Design review of the part shown in the three views and the two pictorial views. Dimensions are in mm from the part's minimum x, y and z. A direction names the side the tool comes from. Give positions to 0.01 mm unless a question says otherwise; leave off trailing zeros. Order: outer loops, then holes, each group sorted by start corner. A loop starts at its lowest first (then second) coordinate and runs counter-clockwise, first axis right, second up.
Item 1: Consider section B-B (x = 10.75). Give the boundary of the cut face in (y, z), plus the area to 3 significant figures.
Item 2: For P1, Ø1.9, axis at x = 7.5, z = 6, coming from the -Y side, flat-tipped, find the tip position at first contact; note if it passes through.
Item 3: The part is to be moulded in two halves that separate along X. For the marked faces 1, 2 and 3, say which applies: released by +X, released by -X, zero draft, split by the parting line, or undercut.
Item 4: Machinability: for the marked faces 4 and 5, which of the approach directions +Z, -Z, +X, -X, +Y, -Y give a long, thin tool a straight path to every point of the face, cutting with its end or side? Answer none if there is none.
Item 5: For probe 1 along Y at (x, z) = (10.5, 4.5); probe 2 along X at (y, z) = (5.5, 6); probe 3 along Y at (x, z) = (7.75, 3.25), list the stretches that pass through material, from the lowest coordinate up.
Item 6: Consider section D-D (x = 5.5). Give the boundary of the cut face in (y, z) (1 decimal).
Item 7: Consider section C-C (y = 2). Give the boundary of the cut face in (x, z), plus the area to 3 significant figures.
Item 8: Consider section A-A (z = 6). Give the boundary of the cut face in (x, y) (1 decimal).
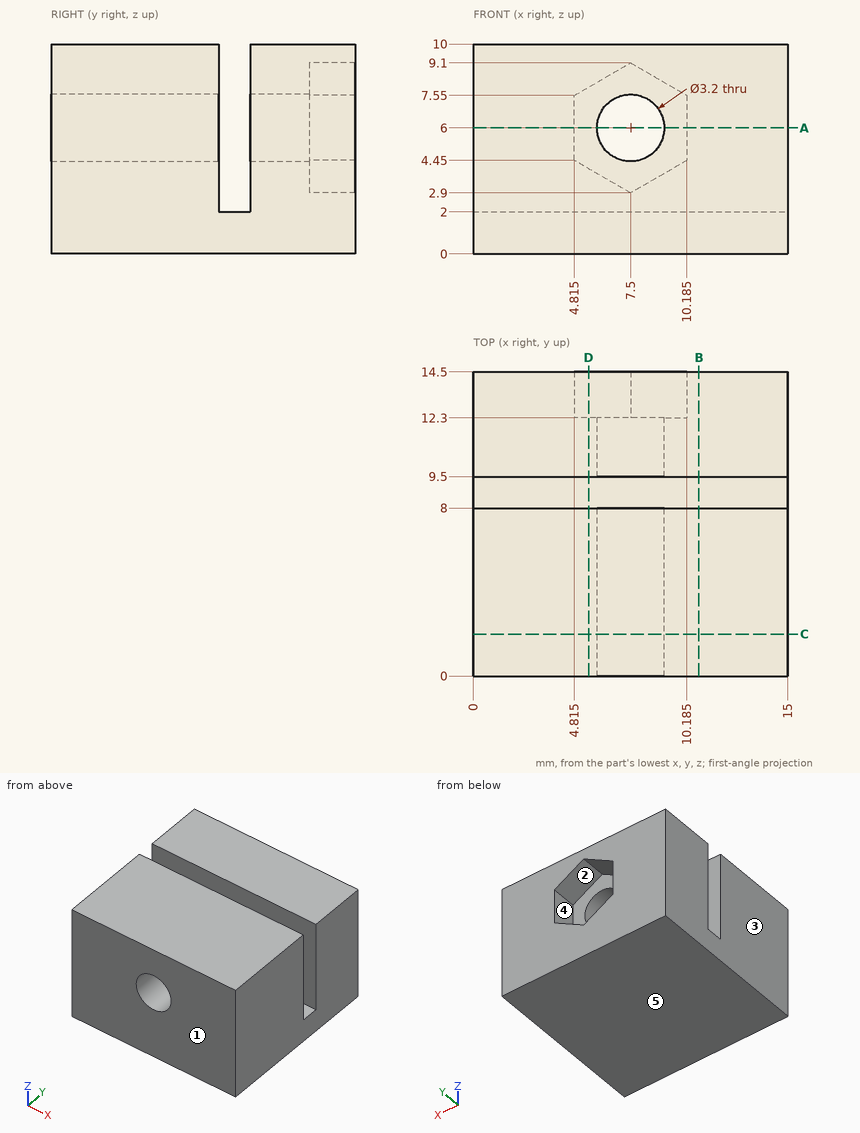
Resolved:
1. outline: (0, 0) - (14.5, 0) - (14.5, 10) - (9.5, 10) - (9.5, 2) - (8, 2) - (8, 10) - (0, 10) - close
1. area: 133 mm2
2. P1: passes through
3. face 1: zero draft
3. face 2: undercut
3. face 3: released by -X
4. face 4: +Y
4. face 5: -Z, +X, -X, +Y, -Y
5. probe 1: y = 0 to 8, 9.5 to 14.5
5. probe 2: x = 0 to 5.9, 9.1 to 15
5. probe 3: y = 0 to 8, 9.5 to 12.3
6. outline: (0, 0) - (14.5, 0) - (14.5, 4.1) - (12.3, 4.1) - (12.3, 7.9) - (14.5, 7.9) - (14.5, 10) - (9.5, 10) - (9.5, 2) - (8, 2) - (8, 10) - (0, 10) - close
7. outline: (0, 0) - (15, 0) - (15, 10) - (0, 10) - close; hole circle Ø3.2 at (7.5, 6)
7. area: 142 mm2
8. outline: (0, 0) - (5.9, 0) - (5.9, 8) - (0, 8) - close; (0, 9.5) - (5.9, 9.5) - (5.9, 12.3) - (4.8, 12.3) - (4.8, 14.5) - (0, 14.5) - close; (9.1, 0) - (15, 0) - (15, 8) - (9.1, 8) - close; (9.1, 9.5) - (15, 9.5) - (15, 14.5) - (10.2, 14.5) - (10.2, 12.3) - (9.1, 12.3) - close
